Check sheet for the modelled part. Datum: model origin and axes. Units: mm. A direction names the side the tool comes from. Coordinates: 2 decimals unless noted, no trailing zeros. Write each loop counter-clockwise with the first axis right and the second up, starting at its lowest first coordinate (ties: lowest second). Pieces come first, ordered by that corner, then holes. Notation, with made-up numbers: (-33, 48) -> (1, 48) arc R16 ccw to (1, 71) -> close; hole circle Ø7 at (53.25, -13.75). An arc over 180 degrees is marked (long way). One line per item, written item: value. Start each with the question number.
1) Sectioned sample at C-C on z = -3.5. Enter the section's corners in (x, y), plus the area to 3 significant figures.
2) Sectioned sample at D-D on x = 12. Enter the section's corners in (y, z), plus the area to 3 significant figures.
3) Sectioned sample at B-B on z = -15.5. Enter the section's corners in (x, y).
4) Set-up check for faces 1 (the flat face through (69.38, 17, 25)), 2 (the flat face through (3, 3, -6.35)), 3 (the flat face through (73, 15, 6.35)), 4 (the flat face through (69.38, 17, -25)), 5 (the flat face through (-65, 43.815, 28)): record each of +Z, -Z, +X, -X, +Y, -Y from which the full face is reachable in a straight line by a thin tool's end or side.
5) Scan lines: line 1 along X through (y, z) = (27, -1); line 2 along X through (y, z) = (5, 27); line 3 along Y through (x, z) = (52.5, 2.5). Record each from-to range of solid material in increasing order. Write a range as [from, to].
6) Draft check along Z on faces 6 (the flat face through (-14, 5.08, 0)), 7 (the flat face through (-67.831, 46, 27)), 8 (the flat face through (73, 15, -6.35)), 9 (the flat face through (-59, 26, -23.292)). Enter one of: +Z half, -Z half, draft (parallel to the pull), parting line (faces both ways), or undercut.
7) Gauge pin test, flat ends, axial feed: P1, Ø4, axis at y = 22, z = -24.5, coming from the +X side; P2, Ø3, axis at x = 72.5, y = 20.5, coming from the +Z side; P3, Ø3, axis at x = -72, z = 2, coming from the +Y side. Record the tip position at first contact, or that the pin passes through.
8) Sectioned sample at A-A on y = 11.5. Enter the section's corners in (x, z).
Autodesk Inventor part; units mm, degrees
ref_plane "YZ Plane" through (0, 0, 0) normal (1, 0, 0) x (0, 1, 0)
ref_plane "XZ Plane" through (0, 0, 0) normal (0, 1, 0) x (-1, 0, 0)
ref_plane "XY Plane" through (0, 0, 0) normal (0, 0, 1) x (1, 0, 0)
sketch "Sketch1" plane through (0, 0, 0) normal (0, 1, 0) x (-1, 0, 0)
  line L0 (69.3801, 23.2918) -> (-69.3801, 23.2918)
  line L1 (-69.3801, 23.2918) -> (-69.3801, -23.2918)
  line L2 (-69.3801, -23.2918) -> (69.3801, -23.2918)
  line L3 (69.3801, -23.2918) -> (69.3801, 23.2918)
  line L4 (69.3801, 23.2918) -> (-69.3801, -23.2918) construction
  line L5 (-69.3801, 23.2918) -> (69.3801, -23.2918) construction
  line L6 (69.3801, -6.35) -> (-69.3801, -6.35)
  line L7 (-69.3801, -6.35) -> (-69.3801, 6.35)
  line L8 (-69.3801, 6.35) -> (69.3801, 6.35)
  line L9 (69.3801, 6.35) -> (69.3801, -6.35)
  line L10 (69.3801, -6.35) -> (-69.3801, 6.35) construction
  line L11 (-69.3801, -6.35) -> (69.3801, 6.35) construction
  line L12 (-62.7307, -31.75) -> (-69.3801, -31.75)
  line L13 (-69.3801, -31.75) -> (-69.3801, 31.75)
  line L14 (-69.3801, 31.75) -> (-62.7307, 31.75)
  line L15 (-62.7307, 31.75) -> (-62.7307, -31.75)
  line L16 (-62.7307, -31.75) -> (-69.3801, 31.75) construction
  line L17 (-69.3801, -31.75) -> (-62.7307, 31.75) construction
  line L18 (-69.3801, 0) -> (61.4807, 0)
  line L19 (61.4807, 0) -> (-69.3801, 0)
  line L20 (55.9943, 31.75) -> (55.9943, -31.75)
  line L21 (55.9943, -31.75) -> (61.4807, -31.75)
  line L22 (61.4807, -31.75) -> (61.4807, 31.75)
  line L23 (61.4807, 31.75) -> (55.9943, 31.75)
  line L24 (55.9943, 31.75) -> (61.4807, -31.75) construction
  line L25 (55.9943, -31.75) -> (61.4807, 31.75) construction
  point P0 (0, 0)
  point P1 (-66.0554, 0)
  point P2 (58.7375, 0)
  dimension "d0" = 138.7602
  dimension "d1" = 46.5836
  dimension "d2" = 12.7
  dimension "d3" = 130.8608
extrude "Extrusion1" add sketch "Sketch1" along normal blind 5.08 contours L22 L8 L20 L0 | L0 L20 L23 L22 | L3 L6 L22 L8 | L22 L18 L20 L8 | L15 L8 L1 L0 | L0 L13 L14 L15 | L20 L18 L15 L8 | L22 L6 L20 L18 | L22 L2 L20 L6 | L15 L18 L1 L8 | L20 L6 L15 L18 | L22 L21 L20 L2 | L15 L6 L1 L18 | L15 L2 L1 L6 | L15 L12 L13 L2
sketch "Sketch2" plane through (0, 5.08, 0) normal (0, 1, 0) x (1, 0, 0)
  point P0 (0, 0)
sketch "Sketch3" plane through (0, 0, 0) normal (0, -1, 0) x (1, 0, 0)
  line L0 (-69.3801, 6.35) -> (-61.4807, 6.35)
  line L1 (-69.3801, 6.35) -> (-75.7301, 6.35)
  line L2 (-75.7301, 6.35) -> (-75.7301, -6.35)
  line L3 (-75.7301, -6.35) -> (-69.3801, -6.35)
  line L4 (-69.3801, -6.35) -> (-69.3801, 6.35)
  line L5 (69.3801, 31.75) -> (69.3801, -31.75)
  line L6 (69.3801, 6.35) -> (75.7301, 6.35)
  line L7 (75.7301, 6.35) -> (75.7301, -6.35)
  line L8 (75.7301, -6.35) -> (69.3801, -6.35)
  line L9 (69.3801, -6.35) -> (69.3801, 6.35)
  point P0 (0, 0)
  dimension "d6" = 6.35
  dimension "d7" = 6.35
extrude "Extrusion2" add sketch "Sketch3" against normal blind 30.48
sketch "Sketch4" plane through (0, 5.08, 0) normal (0, 1, 0) x (1, 0, 0)
  line L0 (-69.3801, -23.2918) -> (69.3801, -23.2918)
  line L1 (69.3801, -23.2918) -> (69.3801, 23.2918)
  line L2 (69.3801, 23.2918) -> (-69.3801, 23.2918)
  line L3 (-69.3801, 23.2918) -> (-69.3801, -23.2918)
  line L4 (-69.3801, -23.2918) -> (69.3801, 23.2918) construction
  line L5 (69.3801, -23.2918) -> (-69.3801, 23.2918) construction
  line L6 (62.7307, 31.75) -> (62.7307, 6.35)
  line L7 (69.3801, 23.2918) -> (62.7307, 23.2918)
  line L8 (62.7307, 23.2918) -> (62.7307, 31.75)
  line L9 (62.7307, 31.75) -> (69.3801, 31.75)
  line L10 (69.3801, 31.75) -> (69.3801, 23.2918)
  line L11 (62.7307, -6.35) -> (62.7307, -31.75)
  line L12 (62.7307, -23.2918) -> (69.3801, -23.2918)
  line L13 (69.3801, -23.2918) -> (69.3801, -31.75)
  line L14 (69.3801, -31.75) -> (62.7307, -31.75)
  line L15 (62.7307, -31.75) -> (62.7307, -23.2918)
  line L16 (-61.4807, -31.75) -> (-55.9943, -31.75)
  line L17 (-61.4807, -6.35) -> (-61.4807, -31.75)
  line L18 (-55.9943, -31.75) -> (-61.4807, -31.75)
  line L19 (-61.4807, -31.75) -> (-61.4807, -23.2918)
  line L20 (-61.4807, -23.2918) -> (-55.9943, -23.2918)
  line L21 (-55.9943, -23.2918) -> (-55.9943, -31.75)
  line L22 (-61.4807, 31.75) -> (-61.4807, 6.35)
  line L23 (-55.9943, 31.75) -> (-61.4807, 31.75)
  line L24 (-61.4807, 23.2918) -> (-55.9943, 23.2918)
  line L25 (-55.9943, 23.2918) -> (-55.9943, 31.75)
  line L26 (-55.9943, 31.75) -> (-61.4807, 31.75)
  line L27 (-61.4807, 31.75) -> (-61.4807, 23.2918)
  point P0 (0, 0)
  dimension "d10" = 138.7602
  dimension "d11" = 46.5836
extrude "Extrusion3" add sketch "Sketch4" along normal blind 42.545 contours L0 L21 L16 L17 | L22 L23 L25 L2 | L0 L13 L14 L11 | L6 L9 L10 L2
sketch "Sketch5" plane through (69.3801, 0, -6.35) normal (1, 0, 0) x (0, 0, -1)
  line L0 (25.4, 47.625) -> (16.9418, 47.625)
  line L1 (25.4, 0) -> (25.4, 47.625)
  line L2 (16.9418, 47.625) -> (25.4, 47.625)
  line L3 (25.4, 47.625) -> (25.4, 43.815)
  line L4 (25.4, 43.815) -> (16.9418, 43.815)
  line L5 (16.9418, 43.815) -> (16.9418, 47.625)
  line L6 (-38.1, 0) -> (-38.1, 47.625)
  line L7 (-29.6418, 5.08) -> (-29.6418, 47.625)
  line L8 (-38.1, 47.625) -> (-29.6418, 47.625)
  line L9 (-29.6418, 47.625) -> (-29.6418, 43.815)
  line L10 (-29.6418, 43.815) -> (-38.1, 43.815)
  line L11 (-38.1, 43.815) -> (-38.1, 47.625)
  point P0 (-6.35, 0)
  dimension "d14" = 3.81
extrude "Extrusion4" add sketch "Sketch5" along normal blind 6.35
sketch "Sketch6" plane through (-61.4807, 0, -31.75) normal (-1, 0, 0) x (0, 0, 1)
  line L0 (0, 0) -> (0, 47.625)
  line L1 (8.4582, 5.08) -> (8.4582, 47.625)
  line L2 (0, 47.625) -> (8.4582, 47.625)
  line L3 (8.4582, 47.625) -> (8.4582, 43.815)
  line L4 (8.4582, 43.815) -> (0, 43.815)
  line L5 (0, 43.815) -> (0, 47.625)
  line L6 (55.0418, 5.08) -> (55.0418, 47.625)
  line L7 (63.5, 0) -> (63.5, 47.625)
  line L8 (55.0418, 47.625) -> (63.5, 47.625)
  line L9 (63.5, 47.625) -> (63.5, 43.815)
  line L10 (63.5, 43.815) -> (55.0418, 43.815)
  line L11 (55.0418, 43.815) -> (55.0418, 47.625)
  point P0 (31.75, 0)
  dimension "d17" = 3.81
extrude "Extrusion5" add sketch "Sketch6" along normal blind 6.35
properties part number "BatteryHanger"
Answers:
1. outline: (-75.73, 0) -> (75.73, 0) -> (75.73, 30.48) -> (69.38, 30.48) -> (69.38, 5.08) -> (-69.38, 5.08) -> (-69.38, 30.48) -> (-75.73, 30.48) -> close
1. area: 1,090 mm2
2. outline: (0, -6.35) -> (5.08, -6.35) -> (5.08, 6.35) -> (0, 6.35) -> close
2. area: 64.5 mm2
3. outline: (-61.48, 0) -> (-55.99, 0) -> (-55.99, 5.08) -> (-61.48, 5.08) -> close; (62.73, 0) -> (69.38, 0) -> (69.38, 5.08) -> (62.73, 5.08) -> close
4. face 1: +Z, +X, -Y
4. face 2: -Z, +Y, -Y
4. face 3: +Z, +X, +Y, -Y
4. face 4: -Z, +X, -Y
4. face 5: +Z, -Z, -X, -Y
5. line 1: x = [-75.73, -69.38], [69.38, 75.73]
5. line 2: x = [-61.48, -55.99], [62.73, 69.38]
5. line 3: y = [0, 5.08]
6. face 6: undercut
6. face 7: draft
6. face 8: -Z half
6. face 9: undercut
7. P1: stops at x = 69.38
7. P2: stops at z = 6.35
7. P3: stops at y = 30.48
8. outline: (-75.73, -6.35) -> (-69.38, -6.35) -> (-69.38, 6.35) -> (-75.73, 6.35) -> close; (-61.48, -31.75) -> (-55.99, -31.75) -> (-55.99, -23.29) -> (-61.48, -23.29) -> close; (-61.48, 23.29) -> (-55.99, 23.29) -> (-55.99, 31.75) -> (-61.48, 31.75) -> close; (62.73, -31.75) -> (69.38, -31.75) -> (69.38, -23.29) -> (62.73, -23.29) -> close; (62.73, 23.29) -> (69.38, 23.29) -> (69.38, 31.75) -> (62.73, 31.75) -> close; (69.38, -6.35) -> (75.73, -6.35) -> (75.73, 6.35) -> (69.38, 6.35) -> close
